```python
from build123d import *

# Parameters (mm, degrees)
F0_R     = 6.35
F1_DEPTH = 2.54
F2_R     = 1.26999


# Not quite as in the source:
# - a fillet or chamfer is up to 0.001 mm smaller than in the source, because OpenCascade refuses the exact size


with BuildPart() as f1:
    # F0 (on Front) → F1 (new body)
    with BuildSketch(Plane.XZ):
        Polygon((8.1817057439, -8.042901042), (11.0273133855, -2.8538767742), (11.0562094944, 3.0641144995), (7.9851864785, 8.1229951402), (2.8745037505, 11.1070155415), (-3.042126907, 10.9768719144), (-8.1817057439, 8.042901042), (-11.0273133855, 2.8538767742), (-11.0562094944, -3.0641144995), (-7.9851864785, -8.1229951402), (-2.8745037505, -11.1070155415), (3.042126907, -10.9768719144), align=None)
        Circle(F0_R, mode=Mode.SUBTRACT)
        with BuildLine():
            Line((-3.042126907, 10.9768719144), (2.8745037505, 11.1070155415))
            Line((2.8745037505, 11.1070155415), (0.1476963834, 12.6991411433))
            ThreePointArc((0.1476963834, 12.6991411433), (0.0620102654, 12.6998486104), (-0.0236786756, 12.699977926))
            Line((-0.0236786756, 12.699977926), (-3.042126907, 10.9768719144))
        make_face()
        with BuildLine():
            Line((-8.1817057439, 8.042901042), (-3.042126907, 10.9768719144))
            Line((-3.042126907, 10.9768719144), (-6.5169336782, 10.9004392312))
            ThreePointArc((-6.5169336782, 10.9004392312), (-6.5903320193, 10.8562205152), (-6.6634303404, 10.8115075775))
            Line((-6.6634303404, 10.8115075775), (-8.1817057439, 8.042901042))
        make_face()
        with BuildLine():
            Line((-11.0273133855, 2.8538767742), (-8.1817057439, 8.042901042))
            Line((-8.1817057439, 8.042901042), (-10.9239306447, 6.4774793917))
            ThreePointArc((-10.9239306447, 6.4774793917), (-10.9673863881, 6.4036267703), (-11.0103428492, 6.3294826284))
            Line((-11.0103428492, 6.3294826284), (-11.0273133855, 2.8538767742))
        make_face()
        with BuildLine():
            Line((-12.6947553855, -0.3649461623), (-11.0562094944, -3.0641144995))
            Line((-11.0562094944, -3.0641144995), (-11.0273133855, 2.8538767742))
            Line((-11.0273133855, 2.8538767742), (-12.6985241258, -0.1936105045))
            ThreePointArc((-12.6985241258, -0.1936105045), (-12.6969287649, -0.2792846905), (-12.6947553855, -0.3649461623))
        make_face()
        with BuildLine():
            Line((-10.9866641736, -6.3704952976), (-7.9851864785, -8.1229951402))
            Line((-7.9851864785, -8.1229951402), (-11.0562094944, -3.0641144995))
            Line((-11.0562094944, -3.0641144995), (-11.0716270281, -6.2216617516))
            ThreePointArc((-11.0716270281, -6.2216617516), (-11.0293966535, -6.2962218401), (-10.9866641736, -6.3704952976))
        make_face()
        with BuildLine():
            Line((-6.0313250452, -11.1764537399), (-2.8745037505, -11.1070155415))
            Line((-2.8745037505, -11.1070155415), (-7.9851864785, -8.1229951402))
            Line((-7.9851864785, -8.1229951402), (-6.1815904476, -11.0940497357))
            ThreePointArc((-6.1815904476, -11.0940497357), (-6.1065967456, -11.1355052057), (-6.0313250452, -11.1764537399))
        make_face()
        with BuildLine():
            Line((0.0236786756, -12.699977926), (3.042126907, -10.9768719144))
            Line((3.042126907, -10.9768719144), (-2.8745037505, -11.1070155415))
            Line((-2.8745037505, -11.1070155415), (-0.1476963834, -12.6991411433))
            ThreePointArc((-0.1476963834, -12.6991411433), (-0.0620102654, -12.6998486104), (0.0236786756, -12.699977926))
        make_face()
        with BuildLine():
            Line((6.6634303404, -10.8115075775), (8.1817057439, -8.042901042))
            Line((8.1817057439, -8.042901042), (3.042126907, -10.9768719144))
            Line((3.042126907, -10.9768719144), (6.5169336782, -10.9004392312))
            ThreePointArc((6.5169336782, -10.9004392312), (6.5903320193, -10.8562205152), (6.6634303404, -10.8115075775))
        make_face()
        with BuildLine():
            ThreePointArc((10.9239306447, -6.4774793917), (10.9673863881, -6.4036267703), (11.0103428492, -6.3294826284))
            Line((11.0103428492, -6.3294826284), (11.0273133855, -2.8538767742))
            Line((11.0273133855, -2.8538767742), (8.1817057439, -8.042901042))
            Line((8.1817057439, -8.042901042), (10.9239306447, -6.4774793917))
        make_face()
        with BuildLine():
            Line((11.0273133855, -2.8538767742), (12.6985241258, 0.1936105045))
            ThreePointArc((12.6985241258, 0.1936105045), (12.6969287649, 0.2792846905), (12.6947553855, 0.3649461623))
            Line((12.6947553855, 0.3649461623), (11.0562094944, 3.0641144995))
            Line((11.0562094944, 3.0641144995), (11.0273133855, -2.8538767742))
        make_face()
        with BuildLine():
            Line((11.0562094944, 3.0641144995), (11.0716270281, 6.2216617516))
            ThreePointArc((11.0716270281, 6.2216617516), (11.0293966535, 6.2962218401), (10.9866641736, 6.3704952976))
            Line((10.9866641736, 6.3704952976), (7.9851864785, 8.1229951402))
            Line((7.9851864785, 8.1229951402), (11.0562094944, 3.0641144995))
        make_face()
        with BuildLine():
            Line((2.8745037505, 11.1070155415), (7.9851864785, 8.1229951402))
            Line((7.9851864785, 8.1229951402), (6.1815904476, 11.0940497357))
            ThreePointArc((6.1815904476, 11.0940497357), (6.1065967456, 11.1355052057), (6.0313250452, 11.1764537399))
            Line((6.0313250452, 11.1764537399), (2.8745037505, 11.1070155415))
        make_face()
    extrude(amount=F1_DEPTH)

    # F2 (radius 1.27 in the source; OpenCascade refuses exactly that, so slightly less here)
    f2_edges = [f1.edges().sort_by_distance(p)[0] for p in [
        (-6.35, -2.54, 0),
        (-6.35, 0, 0),
    ]]
    fillet(f2_edges, radius=F2_R)


solid = f1.part
```
Verification items for the finished model (mm, model axes). Give positions to 0.01 mm unless a question says otherwise; leave off trailing zeros. Order: outer loops, then holes, each group sorted by start corner. A loop starts at its lowest first (then second) coordinate and runs counter-clockwise, first axis right, second up. Notation, with made-up numbers: M -28.75,7 L 9.25,7 A16 ccw 9.25,26 Z; hole C 39.25,-0.75 d11. An arc over 180 degrees is marked long. Return JSON: item names as keys, results as strings. Group by question number.
1) Scan lines: line 1 (Z direction, x = 0, y = -1.3); line 2 (Z direction, x = 4.5, y = -1.15); line 3 (X direction, y = -2.15, z = 4.5). Record each from-to range of solid material in increasing order.
2) Mould release check, pull along X, two halves, no side actions. Record for faces 1 (the face through (-9.534, -1.252, 7.271)), 2 (the face through (5.5, -2.54, -5.5)), 3 (the face through (7.096, -1.252, 9.588)): pulls with the +X half, pulls with the -X half, needs draft (parallel to the pull), parting line crosses it, or undercut.
3) Go/stop test with flat-tipped pins: pin 1 Ø1.5 at (y, z) = (-1, 8.5) entering from +X; pin 2 Ø1 at (x, y) = (10, -1.5) entering from +Z; pin 3 Ø1 at (x, y) = (-6.5, -1) entering from -Z. Record where each tip stops, or that it passes through.
4) Section check B-B on x = -8.5. Record the cut outline in (y, z), and give its area (3 significant figures).
5) Section check A-A on z = -10.25. Record the cut outline in (x, y).
Answer block:
{
 "1": {"line 1": "z = -12.7 to -6.35, 6.35 to 12.7", "line 2": "z = -10.94 to -4.49, 4.49 to 11.14", "line 3": "x = -11.02 to -4.97, 4.97 to 11.06"},
 "2": {"face 1": "pulls with the -X half", "face 2": "needs draft", "face 3": "pulls with the +X half"},
 "3": {"pin 1": "stops at x = 8.62", "pin 2": "stops at z = 7.24", "pin 3": "stops at z = -11.18"},
 "4": {"outline": "M -2.54,-7.82 L 0,-7.82 L 0,7.86 L -2.54,7.86 Z", "area": "39.8 mm^2"},
 "5": {"outline": "M -6.69,-2.54 L 6.97,-2.54 L 6.97,0 L -6.69,0 Z"}
}
